Read the model definition and answer for the solid it produces. Units are mm, in the model's axes. A direction names the side the tool comes from. Give positions to 0.01 mm unless a question says otherwise; leave off trailing zeros. Order: outer loops, then holes, each group sorted by start corner. A loop starts at its lowest first (then second) coordinate and runs counter-clockwise, first axis right, second up. Notation, with made-up numbers: (-20, 59) - (-6, 59) arc R4 cw to (-6, 65) - close; hole circle Ø7 at (48.5, -1.75). An arc over 180 degrees is marked (long way). Write item = value, one per line.
```python
from build123d import *

# Parameters (mm, degrees)
SKETCH1_R           = 3.25
SKETCH1_R_2         = 4.25
SKETCH1_R_3         = 11.25
SKETCH1_R_4         = 1.75
SKETCH1_R_5         = 12
BOSS_EXTRUDE1_DEPTH = 10
FILLET1_R           = 5
SKETCH2_R           = 3
CUT_EXTRUDE1_DEPTH  = 10


with BuildPart() as part:
    # Sketch1 → Boss-Extrude1 (new body)
    with BuildSketch(Plane(origin=(0, 0, 0), x_dir=(1, 0, 0), z_dir=(0, 1, 0))):
        with BuildLine():
            Line((0, -8.25), (50, -8.25))
            Line((50, -8.25), (86.069806885, 8.569627179))
            ThreePointArc((86.069806885, 8.569627179), (88.655178681, 11.391065397), (88.488254512, 15.214257423))
            Line((88.488254512, 15.214257423), (75.387088398, 43.309798821))
            ThreePointArc((75.387088398, 43.309798821), (72.968640771, 45.728246447), (69.561454237, 46.026336644))
            Line((69.561454237, 46.026336644), (45, 39.445114816))
            Line((45, 39.445114816), (45, 60))
            Line((45, 60), (30, 60))
            Line((30, 60), (20.677212951, 37.476864391))
            Line((20.677212951, 37.476864391), (-6.319866656, 5.30299778))
            ThreePointArc((-6.319866656, 5.30299778), (-7.477039243, -3.486600659), (0, -8.25))
        make_face()
        with Locations(Location((0, 0, 0), (0, 0, 270))):
            Circle(SKETCH1_R, mode=Mode.SUBTRACT)
        with Locations(Location((30, 30, 0), (0, 0, 270))):
            Circle(SKETCH1_R_2, mode=Mode.SUBTRACT)
        with Locations(Location((63.358361821, 20.598353756, 0), (0, 0, 270))):
            Circle(SKETCH1_R_3, mode=Mode.SUBTRACT)
        with Locations(Location((42.760008064, 28.095541398, 0), (0, 0, 270))):
            Circle(SKETCH1_R_4, mode=Mode.SUBTRACT)
        with Locations(Location((70.855549463, 41.196707512, 0), (0, 0, 270))):
            Circle(SKETCH1_R_4, mode=Mode.SUBTRACT)
        with Locations(Location((83.956715577, 13.101166114, 0), (0, 0, 270))):
            Circle(SKETCH1_R_4, mode=Mode.SUBTRACT)
        with Locations(Location((55.861174178, 0, 0), (0, 0, 270))):
            Circle(SKETCH1_R_4, mode=Mode.SUBTRACT)
        with Locations(Location((22, 9, 0), (0, 0, 270))):
            Circle(SKETCH1_R_5, mode=Mode.SUBTRACT)
    extrude(amount=BOSS_EXTRUDE1_DEPTH)

    # Fillet1
    fillet1_edges = [part.edges().sort_by_distance(p)[0] for p in [
        (45, 5, -39.445114816),
    ]]
    fillet(fillet1_edges, radius=FILLET1_R)

    # Sketch2 → Cut-Extrude1 (cut)
    with BuildSketch(Plane(origin=(45, 0, 0), x_dir=(0, 0, -1), z_dir=(1, 0, 0))):
        with Locations((55, 5)):
            Circle(SKETCH2_R)
    extrude(amount=-CUT_EXTRUDE1_DEPTH, mode=Mode.SUBTRACT)


solid = part.part
```
1. Section B-B (y = 4) is taken. Count the separate pieces of the cut face and the enclosed holes in it, and give its area (3 significant figures).
Recorded:
separate_pieces = 1
enclosed_holes = 8
area = 3,050 mm^2
2. Straight lines are drawn through the part: L1, parallel to Y at x = 38.5, z = -55; L2, parallel to X at y = 6, z = -11; L3, parallel to X at y = 3, z = -28.5. For each, find the intervals that lie inside material, in ascending order. Write a range as [from, to].
Recorded:
L1 = [0, 2], [8, 10]
L2 = [-1.54, 10.17], [33.83, 57.49], [69.23, 88.49]
L3 = [13.14, 26.02], [33.98, 41.06], [44.46, 55.35], [71.37, 82.29]
3. Section C-C (z = -51) is taken. Determine the outline of the cut face in (x, y), and give its area (3 significant figures).
Recorded:
outline = (26.27, 0) - (45, 0) - (45, 10) - (26.27, 10) - close
area = 187 mm^2
4. For faces 5 (the face through (85.43, 4.93, -12.16)), 6 (the face through (40, 5, -52)), 7 (the face through (60.556, 4.93, -43.613)), determine the directions among +Z, -Z, +X, -X, +Y, -Y from which every point of the face is accessible in a straight line to the end or side of a thin tool.
Recorded:
face_5 = +Y, -Y
face_6 = +X
face_7 = -Z, +Y, -Y
5. Section A-A (x = 22) is taken. Determine the outline of the cut face in (y, z).
Recorded:
outline = (0, -40.67) - (10, -40.67) - (10, -21) - (0, -21) - close; (0, 3) - (10, 3) - (10, 8.25) - (0, 8.25) - close
6. Determine the mould class of faces 1 (the face through (67.78, 4.93, -0.04)), 2 (the face through (7.37, 4.93, -21.62)), 3 (the face through (38, 5, -60)), 4 (the face through (30.187, 4.93, -34.246)) for opening direction X: +X half, -X half, draft (parallel to the pull), parting line (faces both ways), or undercut.
Recorded:
face_1 = +X half
face_2 = -X half
face_3 = draft
face_4 = undercut
7. Flat-ended cylindrical pins translate along their axes: pin 1 (2 mm diameter, centred on x = 60.5, y = 1.5, fed in from -Z); pin 2 (6 mm diameter, centred on y = 3, z = -46.5, fed in from +X); pin 3 (3 mm diameter, centred on y = 2.5, z = -49, fed in from -X). Find the tip coordinate at first contact, or state that the pin passes through.
Recorded:
pin_1 = -43.87
pin_2 = 75.29
pin_3 = 24.83
